Input: part model. Units: mm. Frame: model coordinates. A direction names the side the tool comes from. Give positions to 0.01 mm unless a question says otherwise; leave off trailing zeros. Write each loop counter-clockwise with the first axis right and the second up, starting at its lowest first coordinate (ties: lowest second). Pieces come first, ordered by that corner, then holes. Notation, with made-up numbers: (86, 59) - (135, 59) arc R31 cw to (135, 86) - close; hole circle Ø1 at (45.5, 13.25). An arc over 180 degrees is marked (long way). Use a Markdown table: item, result. Add a question column.
1. Section query C-C, the plane y = -7.5. Return loops of the section in (x, z), plus the area to 3 significant figures.
2. Set-up query: faces 5 (the flat face through (-35.996, -8, -2)), 6 (the flat face through (-45, -2.357, -2)), 7 (the cylindrical face through (-37.95, -4.28, -0.04)), 8 (the flat face through (-54.746, -8, -2)). Return all of +Z, -Z, +X, -X, +Y, -Y with unobstructed straight access to the full face (end or side cutting, diameter ignored); none if empty.
3. Section query A-A, the plane z = -1.6. Return loops of the section in (x, y).
4. Section query B-B, the plane x = -27. Return loops of the section in (y, z).
5. Pin query (flat end, axial travel): pin 1 (1 mm diameter, centred on x = -54, y = -2, fed in from -Z); pin 2 (1.8 mm diameter, centred on x = -46, z = -1, fed in from +Y); pin 3 (1 mm diameter, centred on x = -51, z = 0.5, fed in from -Y); pin 4 (1.8 mm diameter, centred on y = -9, z = 1.5, fed in from +X). Return the tip coordinate at first contact, or that it passes through.
6. Mould query, pull axis Y, two halves, no side actions, for faces 1 (the cylindrical face through (-26.54, 8.96, 1.48)), 2 (the flat face through (-37.496, -8, 0)), 3 (the cylindrical face through (-37.924, -11.606, -0.042)), 4 (the flat face through (-45, -13.557, -2)). Classes: released by +Y, released by -Y, zero draft, split by the parting line, or undercut.
7. Section query D-D, the plane z = 1.1. Return loops of the section in (x, y) (3 decimals).
8. Material intervals for probe 1 along X at (y, z) = (-8.25, -2.45); probe 2 along Z at (x, y) = (-29.5, -3); probe 3 along Y at (x, z) = (-27, 1.6), sorted ascending.
```python
from build123d import *

# Parameters (mm, degrees)
CROQUIS1_R              = 1.5
SALIENTE_EXTRUIR1_DEPTH = 3
SALIENTE_EXTRUIR2_START = 3
CROQUIS2_W              = 18.75
CROQUIS2_H              = 11.2
SALIENTE_EXTRUIR2_DEPTH = 3


with BuildPart() as part:
    # Croquis1 → Saliente-Extruir1 (new body)
    with BuildSketch(Plane.XY):
        with BuildLine():
            ThreePointArc((-30.120896804, 5.459799134), (-45.370896804, -0.856957692), (-60.620896804, 5.459799134))
            ThreePointArc((-60.620896804, 5.459799134), (-64.120896804, 8.959799134), (-67.620896804, 5.459799134))
            ThreePointArc((-67.620896804, 5.459799134), (-67.618884854, 5.372400085), (-67.616529597, 5.285009614))
            ThreePointArc((-67.616529597, 5.285009614), (-45.370896804, -16.326653786), (-23.125264011, 5.285009614))
            ThreePointArc((-23.125264011, 5.285009614), (-23.122908754, 5.372400085), (-23.120896804, 5.459799134))
            ThreePointArc((-23.120896804, 5.459799134), (-26.620896804, 8.959799134), (-30.120896804, 5.459799134))
        make_face()
        with BuildLine():
            Line((-53.245896804, -3.856957692), (-45.370896804, -3.856957692))
            Line((-45.370896804, -3.856957692), (-38.995896804, -3.856957692))
            ThreePointArc((-38.995896804, -3.856957692), (-37.935236632, -4.296297521), (-37.495896804, -5.356957692))
            Line((-37.495896804, -5.356957692), (-37.495896804, -10.556957692))
            ThreePointArc((-37.495896804, -10.556957692), (-37.935236632, -11.617617864), (-38.995896804, -12.056957692))
            Line((-38.995896804, -12.056957692), (-53.245896804, -12.056957692))
            Line((-53.245896804, -12.056957692), (-53.245896804, -3.856957692))
        make_face(mode=Mode.SUBTRACT)
        with Locations((-64.120896804, 5.459799134)):
            Circle(CROQUIS1_R, mode=Mode.SUBTRACT)
        with Locations((-26.620896804, 5.459799134)):
            Circle(CROQUIS1_R, mode=Mode.SUBTRACT)
    extrude(amount=SALIENTE_EXTRUIR1_DEPTH)

    # Croquis2 → Saliente-Extruir2 (add)
    with BuildSketch(Plane(origin=(0, 0, 0), x_dir=(-1, 0, 0), z_dir=(0, 0, -1)).offset(SALIENTE_EXTRUIR2_START)):
        with Locations((45.370896804, -7.956957692)):
            Rectangle(CROQUIS2_W, CROQUIS2_H)
        with BuildLine():
            Line((38.995896804, -12.056957692), (53.245896804, -12.056957692))
            Line((53.245896804, -12.056957692), (53.245896804, -3.856957692))
            Line((53.245896804, -3.856957692), (38.995896804, -3.856957692))
            ThreePointArc((38.995896804, -3.856957692), (37.935236632, -4.296297521), (37.495896804, -5.356957692))
            Line((37.495896804, -5.356957692), (37.495896804, -10.556957692))
            ThreePointArc((37.495896804, -10.556957692), (37.935236632, -11.617617864), (38.995896804, -12.056957692))
        make_face(mode=Mode.SUBTRACT)
    extrude(amount=-SALIENTE_EXTRUIR2_DEPTH)


solid = part.part
```
Result sheet:
| question | item | result |
|---|---|---|
| 1 | outline | (-63.12, 0) - (-54.75, 0) - (-54.75, -3) - (-53.25, -3) - (-53.25, 3) - (-63.12, 3) - close; (-37.5, -3) - (-36, -3) - (-36, 0) - (-27.62, 0) - (-27.62, 3) - (-37.5, 3) - close |
| 1 | area | 68.2 mm² |
| 2 | face 5 | -Z, +X, +Y, -Y |
| 2 | face 6 | -Z, +X, -X, +Y |
| 2 | face 7 | +Z, -Z |
| 2 | face 8 | -Z, -X, +Y, -Y |
| 3 | outline | (-54.75, -13.56) - (-36, -13.56) - (-36, -2.36) - (-54.75, -2.36) - close; hole (-53.25, -12.06) - (-39, -12.06) arc R1.5 ccw to (-37.5, -10.56) - (-37.5, -5.36) arc R1.5 ccw to (-39, -3.86) - (-53.25, -3.86) - close |
| 4 | outline | (-6.63, 0) - (4.01, 0) - (4.01, 3) - (-6.63, 3) - close; (6.91, 0) - (8.94, 0) - (8.94, 3) - (6.91, 3) - close |
| 5 | pin 1 | stops at z = -3 |
| 5 | pin 2 | stops at y = -2.36 |
| 5 | pin 3 | stops at y = -15.73 |
| 5 | pin 4 | stops at x = -28.09 |
| 6 | face 1 | released by +Y |
| 6 | face 2 | undercut |
| 6 | face 3 | undercut |
| 6 | face 4 | released by -Y |
| 7 | outline | (-67.621, 5.46) arc R22.255 ccw to (-67.617, 5.285) arc R22.255 ccw to (-23.125, 5.285) arc R22.255 ccw to (-23.121, 5.46) arc R3.5 ccw to (-30.121, 5.46) arc R21.567 cw to (-60.621, 5.46) arc R3.5 ccw to start; hole circle Ø3 at (-64.121, 5.46); hole (-53.246, -12.057) - (-38.996, -12.057) arc R1.5 ccw to (-37.496, -10.557) - (-37.496, -5.357) arc R1.5 ccw to (-38.996, -3.857) - (-53.246, -3.857) - close; hole circle Ø3 at (-26.621, 5.46) |
| 8 | probe 1 | x = -54.75 to -53.25, -37.5 to -36 |
| 8 | probe 2 | z = 0 to 3 |
| 8 | probe 3 | y = -6.63 to 4.01, 6.91 to 8.94 |
